Input: part model. Units: mm. Frame: model coordinates. Face numbers are marked on the shaded views. A direction names the side the tool comes from. Coordinates: 2 decimals unless noted, no trailing zeros. Loops run counter-clockwise (first coordinate to the right, second up) from the corner with the lowest first, then second, coordinate; pieces in that order, holes last. Notation, with made-up numbers: (5, 46) -> (55, 46) arc R19 cw to (55, 60) -> close; hole circle Ø8 at (7, 88). An arc over 180 degrees is marked (long way). Put each result on its own line as item: value. Start each with the question number.
1) Set-up query: the marked faces 1, 2 and 3. Return all of +Z, -Z, +X, -X, +Y, -Y with unobstructed straight access to the full face (end or side cutting, diameter ignored); none if empty.
2) Material intervals for L1, parallel to Y at x = 0, z = 1.9; L2, parallel to Y at x = 14, z = 2.05; L3, parallel to X at y = -17, z = 2, sorted ascending.
3) Contact query for flat-ended pins moving along their axis: P1, Ø4, axis at x = 15.3, y = 15.7, coming from the -Z side; P2, Ø4.5, axis at x = 0, y = 27, coming from the +Z side; P3, Ø2.5, axis at y = -26.5, z = 2, coming from the +X side; P4, Ø1, axis at x = 33, z = 2, coming from the +Y side. Output: stop coordinate, or through.
4) Cut plane B-B (x = 1.5). Return the cut outline in (y, z), plus the area to 3 significant figures.
5) Cut plane C-C (x = 30). Return the cut outline in (y, z).
6) Cut plane D-D (z = 4.1). Return the cut outline in (x, y), plus the area to 3 significant figures.
7) Cut plane A-A (y = -27). Return the cut outline in (x, z), plus the area to 4 significant figures.
from build123d import *

# Parameters (mm, degrees)
SKETCH1_W           = 41
SKETCH1_H           = 70
SKETCH1_R           = 1.55
SKETCH1_R_2         = 2.75
BOSS_EXTRUDE1_DEPTH = 5
CHAMFER1_SIZE       = 5
SKETCH2_W           = 20
SKETCH2_H           = 34.1
SKETCH2_R           = 2.5
BOSS_EXTRUDE2_DEPTH = 5
CHAMFER2_SIZE       = 5


with BuildPart() as part:
    # Sketch1 → Boss-Extrude1 (new body)
    with BuildSketch(Plane.XY):
        Rectangle(SKETCH1_W, SKETCH1_H)
        with Locations((-15.704778157, -15.295221843)):
            Circle(SKETCH1_R, mode=Mode.SUBTRACT)
        with Locations((15.295221843, -15.295221843)):
            Circle(SKETCH1_R, mode=Mode.SUBTRACT)
        with Locations((15.295221843, 15.704778157)):
            Circle(SKETCH1_R, mode=Mode.SUBTRACT)
        with Locations((-15.704778157, 15.704778157)):
            Circle(SKETCH1_R, mode=Mode.SUBTRACT)
        with Locations((0, 27)):
            Circle(SKETCH1_R_2, mode=Mode.SUBTRACT)
        with Locations((0, -27)):
            Circle(SKETCH1_R_2, mode=Mode.SUBTRACT)
    extrude(amount=BOSS_EXTRUDE1_DEPTH)

    # Chamfer1
    chamfer1_edges = [part.edges().sort_by_distance(p)[0] for p in [
        (-20.5, 35, 2.5),
        (20.5, 35, 2.5),
        (20.5, -35, 2.5),
        (-20.5, -35, 2.5),
    ]]
    chamfer(chamfer1_edges, length=CHAMFER1_SIZE)

    # Sketch2 → Boss-Extrude2 (add)
    with BuildSketch(Plane.XY.offset(5)):
        with Locations((30.5, 0.204778157)):
            Rectangle(SKETCH2_W, SKETCH2_H)
        with Locations((30, 0)):
            Circle(SKETCH2_R, mode=Mode.SUBTRACT)
    extrude(amount=-BOSS_EXTRUDE2_DEPTH)

    # Chamfer2
    chamfer2_edges = [part.edges().sort_by_distance(p)[0] for p in [
        (40.5, 17.254778157, 2.5),
        (40.5, -16.845221843, 2.5),
    ]]
    chamfer(chamfer2_edges, length=CHAMFER2_SIZE)


solid = part.part
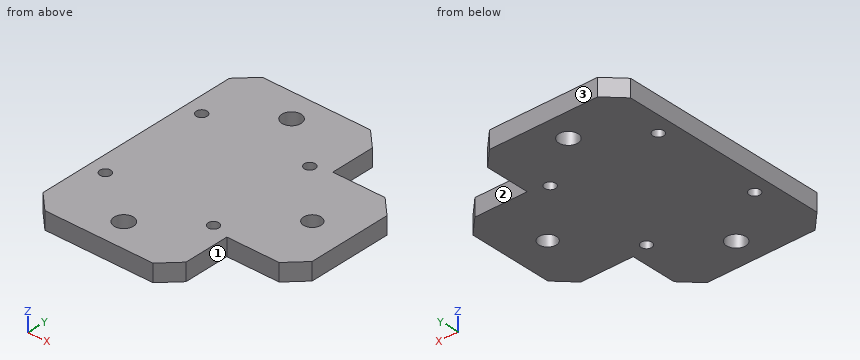
Results found:
1. face 1: +Z, -Z, +X, -Y
1. face 2: +Z, -Z, +X, +Y
1. face 3: +Z, -Z, +X, -X, +Y
2. L1: y = -35 to -29.75, -24.25 to 24.25, 29.75 to 35
2. L2: y = -35 to -16.15, -14.44 to 14.85, 16.56 to 35
2. L3: x = -20.5 to 20.5
3. P1: stops at z = 0
3. P2: passes through
3. P3: stops at x = 20.5
3. P4: stops at y = 17.25
4. outline: (-35, 0) -> (-29.3, 0) -> (-29.3, 5) -> (-35, 5) -> close; (-24.7, 0) -> (24.7, 0) -> (24.7, 5) -> (-24.7, 5) -> close; (29.3, 0) -> (35, 0) -> (35, 5) -> (29.3, 5) -> close
4. area: 304 mm2
5. outline: (-16.85, 0) -> (-2.5, 0) -> (-2.5, 5) -> (-16.85, 5) -> close; (2.5, 0) -> (17.25, 0) -> (17.25, 5) -> (2.5, 5) -> close
6. outline: (-20.5, -30) -> (-15.5, -35) -> (15.5, -35) -> (20.5, -30) -> (20.5, -16.85) -> (35.5, -16.85) -> (40.5, -11.85) -> (40.5, 12.25) -> (35.5, 17.25) -> (20.5, 17.25) -> (20.5, 30) -> (15.5, 35) -> (-15.5, 35) -> (-20.5, 30) -> close; hole circle Ø3.1 at (-15.7, -15.3); hole circle Ø3.1 at (-15.7, 15.7); hole circle Ø5.5 at (0, -27); hole circle Ø5.5 at (0, 27); hole circle Ø3.1 at (15.3, -15.3); hole circle Ø3.1 at (15.3, 15.7); hole circle Ø5 at (30, 0)
6. area: 3,380 mm2
7. outline: (-20.5, 0) -> (-2.75, 0) -> (-2.75, 5) -> (-20.5, 5) -> close; (2.75, 0) -> (20.5, 0) -> (20.5, 5) -> (2.75, 5) -> close
7. area: 177.5 mm2
